```python
from build123d import *

# Parameters (mm, degrees)
CYLINDER1905_R               = 3
CYLINDER1905_DEPTH           = 3
CYLINDER1905_PLACEMENT_ANGLE = 45
CYLINDER1904_R               = 3
CYLINDER1904_DEPTH           = 3
CYLINDER1904_PLACEMENT_ANGLE = 45
CYLINDER1907_R               = 3
CYLINDER1907_DEPTH           = 3
CYLINDER1907_PLACEMENT_ANGLE = 45
CYLINDER1909_R               = 3
CYLINDER1909_DEPTH           = 3
CYLINDER1909_PLACEMENT_ANGLE = 45
CYLINDER1906_R               = 1.5
CYLINDER1906_DEPTH           = 50
CYLINDER1906_PLACEMENT_ANGLE = 45
CYLINDER1908_R               = 1.5
CYLINDER1908_DEPTH           = 50
CYLINDER1908_PLACEMENT_ANGLE = 45
CYLINDER1901_R               = 8
CYLINDER1901_DEPTH           = 6
CYLINDER1900_R               = 1.5
CYLINDER1900_DEPTH           = 50
CYLINDER1900_PLACEMENT_ANGLE = 45
CYLINDER1896_R               = 1.5
CYLINDER1896_DEPTH           = 50
CYLINDER1896_PLACEMENT_ANGLE = 45
BOX800_W                     = 68
BOX800_H                     = 36
BOX800_DEPTH                 = 6


with BuildPart() as obj1:
    # Cylinder1905 → Cylinder1905 (new body)
    with BuildSketch(Plane.XY):
        Circle(CYLINDER1905_R)
    extrude(amount=CYLINDER1905_DEPTH)


with BuildPart() as obj1_1:
    # Cylinder1905 placement: moved
    add(obj1.part.moved(Location((22, 118, 0))).rotate(Axis((22, 118, 0), (0, 0, 1)), CYLINDER1905_PLACEMENT_ANGLE))


with BuildPart() as compound956:
    # Cylinder1904 → Cylinder1904 (new body)
    with BuildSketch(Plane.XY):
        Circle(CYLINDER1904_R)
    extrude(amount=CYLINDER1904_DEPTH)


with BuildPart() as compound956_1:
    # Cylinder1904 placement: moved
    add(compound956.part.moved(Location((-22, 118, 0))).rotate(Axis((-22, 118, 0), (0, 0, 1)), CYLINDER1904_PLACEMENT_ANGLE))

    # Compound956: union obj1
    add(obj1_1.part)


with BuildPart() as compound956_2:
    # Compound956 placement: moved
    add(compound956_1.part.moved(Location((0, 0, 25))))


with BuildPart() as obj2:
    # Cylinder1907 → Cylinder1907 (new body)
    with BuildSketch(Plane.XY):
        Circle(CYLINDER1907_R)
    extrude(amount=CYLINDER1907_DEPTH)


with BuildPart() as obj2_1:
    # Cylinder1907 placement: moved
    add(obj2.part.moved(Location((31, 101, 0))).rotate(Axis((31, 101, 0), (0, 0, 1)), CYLINDER1907_PLACEMENT_ANGLE))


with BuildPart() as compound957:
    # Cylinder1909 → Cylinder1909 (new body)
    with BuildSketch(Plane.XY):
        Circle(CYLINDER1909_R)
    extrude(amount=CYLINDER1909_DEPTH)


with BuildPart() as compound957_1:
    # Cylinder1909 placement: moved
    add(compound957.part.moved(Location((-31, 101, 0))).rotate(Axis((-31, 101, 0), (0, 0, 1)), CYLINDER1909_PLACEMENT_ANGLE))

    # Compound957: union obj2
    add(obj2_1.part)


with BuildPart() as compound957_2:
    # Compound957 placement: moved
    add(compound957_1.part.moved(Location((0, 0, 25))))


with BuildPart() as obj3:
    # Cylinder1906 → Cylinder1906 (new body)
    with BuildSketch(Plane.XY):
        Circle(CYLINDER1906_R)
    extrude(amount=CYLINDER1906_DEPTH)


with BuildPart() as obj3_1:
    # Cylinder1906 placement: moved
    add(obj3.part.moved(Location((22, 118, 0))).rotate(Axis((22, 118, 0), (0, 0, 1)), CYLINDER1906_PLACEMENT_ANGLE))


with BuildPart() as compound958:
    # Cylinder1908 → Cylinder1908 (new body)
    with BuildSketch(Plane.XY):
        Circle(CYLINDER1908_R)
    extrude(amount=CYLINDER1908_DEPTH)


with BuildPart() as compound958_1:
    # Cylinder1908 placement: moved
    add(compound958.part.moved(Location((-22, 118, 0))).rotate(Axis((-22, 118, 0), (0, 0, 1)), CYLINDER1908_PLACEMENT_ANGLE))

    # Compound958: union obj3
    add(obj3_1.part)


with BuildPart() as obj4:
    # Cylinder1901 → Cylinder1901 (new body)
    with BuildSketch(Plane(origin=(0, 83, 25), x_dir=(1, 0, 0), z_dir=(0, 0, 1))):
        Circle(CYLINDER1901_R)
    extrude(amount=CYLINDER1901_DEPTH)


with BuildPart() as obj5:
    # Cylinder1900 → Cylinder1900 (new body)
    with BuildSketch(Plane.XY):
        Circle(CYLINDER1900_R)
    extrude(amount=CYLINDER1900_DEPTH)


with BuildPart() as obj5_1:
    # Cylinder1900 placement: moved
    add(obj5.part.moved(Location((31, 101, 0))).rotate(Axis((31, 101, 0), (0, 0, 1)), CYLINDER1900_PLACEMENT_ANGLE))


with BuildPart() as compound954:
    # Cylinder1896 → Cylinder1896 (new body)
    with BuildSketch(Plane.XY):
        Circle(CYLINDER1896_R)
    extrude(amount=CYLINDER1896_DEPTH)


with BuildPart() as compound954_1:
    # Cylinder1896 placement: moved
    add(compound954.part.moved(Location((-31, 101, 0))).rotate(Axis((-31, 101, 0), (0, 0, 1)), CYLINDER1896_PLACEMENT_ANGLE))

    # Compound954: union obj5
    add(obj5_1.part)


with BuildPart() as cut610:
    # Box800 → Box800 (new body)
    with BuildSketch(Plane(origin=(-34, 86, 25), x_dir=(1, 0, 0), z_dir=(0, 0, 1))):
        with Locations((34, 18)):
            Rectangle(BOX800_W, BOX800_H)
    extrude(amount=BOX800_DEPTH)

    # Cut606: cut Compound954
    add(compound954_1.part, mode=Mode.SUBTRACT)

    # Cut603: cut obj4
    add(obj4.part, mode=Mode.SUBTRACT)

    # Cut609: cut Compound958
    add(compound958_1.part, mode=Mode.SUBTRACT)

    # Cut611: cut Compound957
    add(compound957_2.part, mode=Mode.SUBTRACT)

    # Cut610: cut Compound956
    add(compound956_2.part, mode=Mode.SUBTRACT)


solid = cut610.part
```
Input: part model. Units: mm. Frame: model coordinates. A direction names the side the tool comes from. Round coordinates to 2 decimals unless told otherwise and drop trailing zeros. Loops run counter-clockwise (first coordinate to the right, second up) from the corner with the lowest first, then second, coordinate; pieces in that order, holes last.
1) Pull-direction query (Y, two-part tool) for faces 3 (the flat face through (-20, 118, 28)), 4 (the flat face through (0, 104, 31)), 5 (the cylindrical face through (-22.196, 116.513, 29.479)), 6 (the flat face through (0, 122, 28)); classes: released by +Y, released by -Y, zero draft, split by the parting line, or undercut.
Ans:
face 3: undercut
face 4: zero draft
face 5: undercut
face 6: released by +Y
2) Material intervals for line 1 (X direction, y = 118, z = 27); line 2 (X direction, y = 101, z = 29); line 3 (Y direction, x = -22, z = 26.65), sorted ascending.
Ans:
line 1: x = -34 to -25, -19 to 19, 25 to 34
line 2: x = -34 to -32.5, -29.5 to 29.5, 32.5 to 34
line 3: y = 86 to 115, 121 to 122
3) Set-up query: faces 1 (the cylindrical face through (22, 115, 26)), 2 (the cylindrical face through (-31.196, 99.513, 29.479)). Return all of +Z, -Z, +X, -X, +Y, -Y with unobstructed straight access to the full face (end or side cutting, diameter ignored); none if empty.
Ans:
face 1: -Z
face 2: +Z, -Z
4) Section query A-A on y = 118. Return the cut outline in (x, z).
Ans:
outline: (-34, 25) - (-25, 25) - (-25, 28) - (-23.5, 28) - (-23.5, 31) - (-34, 31) - close; (-20.5, 28) - (-19, 28) - (-19, 25) - (19, 25) - (19, 28) - (20.5, 28) - (20.5, 31) - (-20.5, 31) - close; (23.5, 28) - (25, 28) - (25, 25) - (34, 25) - (34, 31) - (23.5, 31) - close
5) Section query D-D on z = 30.05. Return the cut outline in (x, y).
Ans:
outline: (-34, 86) - (-7.42, 86) arc R8 cw to (7.42, 86) - (34, 86) - (34, 122) - (-34, 122) - close; hole circle Ø3 at (-31, 101); hole circle Ø3 at (-22, 118); hole circle Ø3 at (22, 118); hole circle Ø3 at (31, 101)
6) Pin query (flat end, axial travel): pin 1 (5 mm diameter, centred on x = 31, y = 101, fed in from -Z); pin 2 (2.5 mm diameter, centred on x = 22, y = 118, fed in from -Z); pin 3 (3 mm diameter, centred on x = -5.5, z = 28.5, fed in from -Y). Return the tip coordinate at first contact, or that it passes through.
Ans:
pin 1: stops at z = 28
pin 2: passes through
pin 3: stops at y = 86.87
7) Section query B-B on x = -22. Return the cut outline in (y, z), plus the area to 3 significant figures.
Ans:
outline: (86, 25) - (115, 25) - (115, 28) - (116.5, 28) - (116.5, 31) - (86, 31) - close; (119.5, 28) - (121, 28) - (121, 25) - (122, 25) - (122, 31) - (119.5, 31) - close
area: 189 mm2
